Autodesk Inventor part; units mm, degrees
ref_plane "YZ Plane" through (0, 0, 0) normal (1, 0, 0) x (0, 1, 0)
ref_plane "XZ Plane" through (0, 0, 0) normal (0, 1, 0) x (-1, 0, 0)
ref_plane "XY Plane" through (0, 0, 0) normal (0, 0, 1) x (1, 0, 0)
sketch "Skizze1" plane through (0, 0, 0) normal (0, 0, 1) x (1, 0, 0)
  line L0 (0, 0) -> (35, 0)
  line L1 (35, 0) -> (35, 17.5)
  line L2 (35, 17.5) -> (0, 17.5)
  line L3 (0, 17.5) -> (0, 0)
  dimension "d0" = 35
  dimension "d1" = 17.5
extrude "Extrusion1" add sketch "Skizze1" along normal blind 12.5
sketch "Skizze2" plane through (0, 0, 12.5) normal (0, 0, 1) x (1, 0, 0)
  line L0 (35, 0) -> (35, 17.5)
  line L1 (35, 12.75) -> (5, 12.75)
  line L2 (5, 12.75) -> (5, 4.75)
  line L3 (5, 4.75) -> (35, 4.75)
  line L4 (35, 4.75) -> (35, 12.75)
  line L5 (0, 0) -> (35, 0)
  dimension "d4" = 4.75
  dimension "d5" = 4.75
  dimension "d6" = 30
extrude "Extrusion2" cut sketch "Skizze2" against normal blind 12.5
sketch "Skizze3" plane through (0, 0, 12.5) normal (0, 0, 1) x (1, 0, 0)
  circle A0 centre (0, 17.5) radius 5
  circle A1 centre (0, 0) radius 5
  line L0 (0, 0) -> (35, 0)
  circle A2 centre (30, 0) radius 5
  line L1 (35, 17.5) -> (0, 17.5)
  circle A3 centre (30, 17.5) radius 5
  line L2 (35, 12.75) -> (35, 17.5)
  dimension "d9" = 10
  dimension "d10" = 10
  dimension "d11" = 10
  dimension "d12" = 10
extrude "Extrusion3" cut sketch "Skizze3" against normal blind 12.5
sketch "Skizze4" plane through (0, 0, 12.5) normal (0, 0, 1) x (1, 0, 0)
  circle A0 centre (30, 17.5) radius 5
  circle A1 centre (30, 0.0223) radius 5
  circle A2 centre (0, 0) radius 5
  circle A3 centre (0, 17.5) radius 5
  line L0 (0, 12.5) -> (0, 5)
  line L1 (5, 4.75) -> (5, 12.75)
  dimension "d17" = 10
  dimension "d18" = 10
  dimension "d19" = 10
  dimension "d20" = 10
  dimension "d21" = 30
  dimension "d24" = 25
extrude "Extrusion4" add sketch "Skizze4" against normal blind 12.5
sketch "Skizze5" plane through (0, 0, 12.5) normal (0, 0, 1) x (1, 0, 0)
  arc A0 (25, 0.0111) -> (35, 0.0111) centre (30, 0.0223) ccw
  point P0 (0, 0)
  point P1 (0, 0)
  point P2 (0, 17.5)
  point P3 (30, 17.5223)
  dimension "d27" = 17.5
  dimension "d28" = 17.5
  dimension "d29" = 30
sketch "Skizze6" plane through (0, 0, 12.5) normal (0, 0, 1) x (1, 0, 0)
  point P0 (0, 0)
hole "Bohrung1" at (0, 0, 12.5) at (0, 17.5, 12.5) at (30, 17.5223, 12.5) at (30, 0.0223, 12.5) direction (0, 0, -1) diameter 3 end through all
sketch "Skizze8" plane through (5, 4.75, 12.5) normal (1, 0, 0) x (0, 0, -1)
  line L0 (12.5, 8) -> (12.5, 0)
  line L1 (12.5, 0) -> (0, 0)
  point P0 (12.5, -4.75)
  point P1 (6.25, 3.75)
  dimension "d37" = 6.25
  dimension "d38" = 3.75
hole "Bohrung2" at (5, 8.5, 6.25) direction (-1, 0, 0) diameter 5 end through all
sketch "Skizze9" plane through (5, 4.75, 12.5) normal (1, 0, 0) x (0, 0, -1)
  line L0 (12.5, 0) -> (0, 0)
  line L1 (0, 8) -> (12.5, 8)
  line L2 (0, 0) -> (12.5, 0)
  line L3 (12.5, 0) -> (12.5, 8)
  line L4 (12.5, 8) -> (0, 8)
  line L5 (0, 8) -> (0, 0)
  point P0 (12.5, -4.75)
extrude "Extrusion5" cut sketch "Skizze9" along normal blind 30
properties part number "halterung_arm"
Work out the finished part from the listing and answer in its coordinate system (mm). A direction names the side the tool comes from. Round coordinates to 2 decimals unless told otherwise and drop trailing zeros. Loops run counter-clockwise (first coordinate to the right, second up) from the corner with the lowest first, then second, coordinate; pieces in that order, holes last. Notation, with made-up numbers: M 85,54.25 L 105,54.25 A13 cw 105,67.25 Z; hole C -2.5,17 d8. An arc over 180 degrees is marked long. One line per question, with ' | ' between items. Start each with the question number.
(1) Find the intervals of material crossed by line 1 (Y direction, x = 30, z = 3.5); line 2 (Y direction, x = 17, z = 5); line 3 (X direction, y = 17.75, z = 1), in increasing order.
(2) A cutting plane is placed at C-C on x = 30. Write down the section's boundary in (y, z).
(3) Flat-ended cylindrical pins translate along their axes: pin 1 Ø2 at (y, z) = (4, 7.5) entering from -X; pin 2 Ø4 at (y, z) = (8.5, 5.5) entering from +X; pin 3 Ø3 at (x, z) = (14, 7) entering from -Y; pin 4 Ø2.5 at (x, y) = (30, 17.52) entering from +Z. Find the tip coordinate at first contact, or state that the pin passes through.
(4) A tool of negligible diameter and unlimited length cuts with its end or side. For faces 1 (the face through (0, 11.3, 6.2)), 2 (the face through (20, 12.75, 6)), 3 (the face through (2.46, 10.72, 5.1)), from which of +Z, -Z, +X, -X, +Y, -Y can it reach the whole face along a straight path? Write none if from no direction.
(5) A cutting plane is placed at A-A on z = 6.25. Give the number of separate pieces and of enclosed holes in the cut face, plus the area to 3 significant figures.
(6) A cutting plane is placed at B-B on y = 8.5. Write down the section's boundary in (x, z), plus the area to 3 significant figures.
(7) For a pull along Y with two mould halves and no side action, classify faces 4 (the face through (15, 15, 0)), 5 (the face through (30.1, 22.5, 6.3)), 6 (the face through (-4, -3, 6)), 7 (the face through (15, 0, 6)) as released by +Y, released by -Y, zero draft, split by the parting line, or undercut.
Geometry check:
1) line 1: y = -4.98 to -1.48, 1.52 to 4.75, 12.75 to 16.02, 19.02 to 22.5 | line 2: y = 0 to 4.75, 12.75 to 17.5 | line 3: x = -4.99 to -1.48, 1.48 to 4.99, 25.01 to 28.52, 31.48 to 34.99
2) outline: M -4.98,0 L -1.48,0 L -1.48,12.5 L -4.98,12.5 Z; M 1.52,0 L 4.75,0 L 4.75,12.5 L 1.52,12.5 Z; M 12.75,0 L 16.02,0 L 16.02,12.5 L 12.75,12.5 Z; M 19.02,0 L 22.5,0 L 22.5,12.5 L 19.02,12.5 Z
3) pin 1: stops at x = -4 | pin 2: stops at x = 5 | pin 3: stops at y = 0 | pin 4: passes through
4) face 1: +Z, -Z, -X | face 2: +Z, -Z, +X | face 3: +X, -X
5) separate pieces: 2 | enclosed holes: 4 | area: 515 mm²
6) outline: M 0,0 L 5,0 L 5,3.75 L 0,3.75 Z; M 0,8.75 L 5,8.75 L 5,12.5 L 0,12.5 Z | area: 37.5 mm²
7) face 4: zero draft | face 5: released by +Y | face 6: undercut | face 7: released by -Y
